Read the model definition and answer for the solid it produces. Units are mm, in the model's axes. Coordinates: 2 decimals unless noted, no trailing zeros. Loops run counter-clockwise (first coordinate to the right, second up) from the corner with the lowest first, then second, coordinate; pieces in that order, holes last.
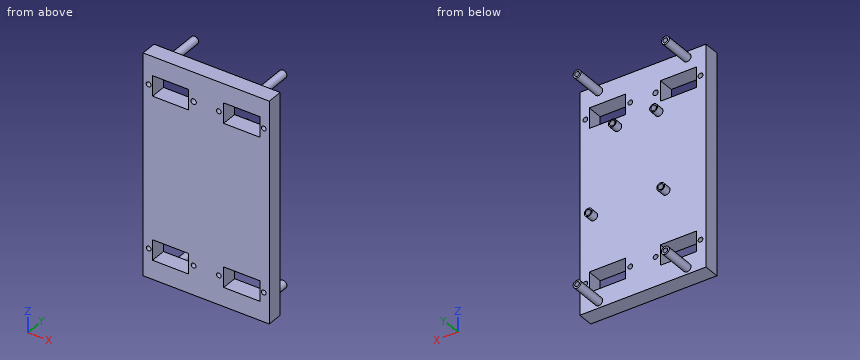
from build123d import *

# Parameters (mm, degrees)
SKETCH1_W           = 80
SKETCH1_H           = 140
BOSS_EXTRUDE1_DEPTH = 10
SKETCH4_W           = 22.9
SKETCH4_H           = 12.9
CUT_EXTRUDE2_DEPTH  = 162.554944214
SKETCH6_R           = 1.5
CUT_EXTRUDE4_DEPTH  = 162.554944214
SKETCH9_W           = 22.9
SKETCH9_H           = 12.9
CUT_EXTRUDE5_DEPTH  = 162.554944214
SKETCH13_R          = 2.5
BOSS_EXTRUDE2_DEPTH = 20
SKETCH14_R          = 1.5
CUT_EXTRUDE8_DEPTH  = 5
SKETCH15_R          = 2.5
BOSS_EXTRUDE3_DEPTH = 20
SKETCH16_R          = 1.5
CUT_EXTRUDE9_DEPTH  = 5
SKETCH17_R          = 1.567331153
SKETCH17_R_2        = 1.710433461
CUT_EXTRUDE10_DEPTH = 163.480768093
SKETCH24_R          = 2.5
BOSS_EXTRUDE5_DEPTH = 5
SKETCH26_R          = 1.8
CUT_EXTRUDE11_DEPTH = 5


with BuildPart() as part:
    # Sketch1 → Boss-Extrude1 (new body)
    with BuildSketch(Plane(origin=(0, 0, 0), x_dir=(1, 0, 0), z_dir=(0, 1, 0))):
        with Locations((-40, 70)):
            Rectangle(SKETCH1_W, SKETCH1_H)
    extrude(amount=BOSS_EXTRUDE1_DEPTH)

    # Sketch4 → Cut-Extrude2 (cut, through all)
    with BuildSketch(Plane(origin=(0, 10, 0), x_dir=(1, 0, 0), z_dir=(0, 1, 0))):
        with Locations((-17.45, 121.55)):
            Rectangle(SKETCH4_W, SKETCH4_H)
    cut_extrude2 = extrude(amount=-CUT_EXTRUDE2_DEPTH, mode=Mode.SUBTRACT)

    # Sketch6 → Cut-Extrude4 (cut, through all)
    with BuildSketch(Plane(origin=(0, 10, 0), x_dir=(1, 0, 0), z_dir=(0, 1, 0))):
        with Locations(Location((-3.5, 121.55, 0), (0, 0, 270))):
            Circle(SKETCH6_R)
        with Locations(Location((-32, 121.55, 0), (0, 0, 270))):
            Circle(SKETCH6_R)
    cut_extrude4 = extrude(amount=-CUT_EXTRUDE4_DEPTH, mode=Mode.SUBTRACT)

    # Mirror4: Cut-Extrude2, Cut-Extrude4 across plane
    add(cut_extrude2.mirror(Plane.XY.offset(-70)), mode=Mode.SUBTRACT)
    add(cut_extrude4.mirror(Plane.XY.offset(-70)), mode=Mode.SUBTRACT)

    # Mirror15: Cut-Extrude2, Cut-Extrude4 across plane
    add(cut_extrude2.mirror(Plane.ZY.offset(40)), mode=Mode.SUBTRACT)
    add(cut_extrude4.mirror(Plane.ZY.offset(40)), mode=Mode.SUBTRACT)

    # Sketch9 → Cut-Extrude5 (cut, through all)
    with BuildSketch(Plane(origin=(0, 10, 0), x_dir=(1, 0, 0), z_dir=(0, 1, 0))):
        with Locations((-62.55, 18.45)):
            Rectangle(SKETCH9_W, SKETCH9_H)
    extrude(amount=-CUT_EXTRUDE5_DEPTH, mode=Mode.SUBTRACT)

    # Sketch13 → Boss-Extrude2 (add)
    with BuildSketch(Plane(origin=(0, 10, 0), x_dir=(1, 0, 0), z_dir=(0, 1, 0))):
        with Locations(Location((-68, 136, 0), (0, 0, 270))):
            Circle(SKETCH13_R)
    boss_extrude2 = extrude(amount=BOSS_EXTRUDE2_DEPTH)

    # Sketch14 → Cut-Extrude8 (cut)
    with BuildSketch(Plane(origin=(0, 30, 0), x_dir=(1, 0, 0), z_dir=(0, 1, 0))):
        with Locations(Location((-68, 136, 0), (0, 0, 270))):
            Circle(SKETCH14_R)
    cut_extrude8 = extrude(amount=-CUT_EXTRUDE8_DEPTH, mode=Mode.SUBTRACT)

    # Sketch15 → Boss-Extrude3 (add)
    with BuildSketch(Plane(origin=(0, 10, 0), x_dir=(1, 0, 0), z_dir=(0, 1, 0))):
        with Locations(Location((-12, 136, 0), (0, 0, 270))):
            Circle(SKETCH15_R)
    boss_extrude3 = extrude(amount=BOSS_EXTRUDE3_DEPTH)

    # Sketch16 → Cut-Extrude9 (cut)
    with BuildSketch(Plane(origin=(0, 30, 0), x_dir=(1, 0, 0), z_dir=(0, 1, 0))):
        with Locations(Location((-12, 136, 0), (0, 0, 270))):
            Circle(SKETCH16_R)
    cut_extrude9 = extrude(amount=-CUT_EXTRUDE9_DEPTH, mode=Mode.SUBTRACT)

    # Mirror22: Boss-Extrude2, Cut-Extrude8, Boss-Extrude3, Cut-Extrude9 across plane
    add(boss_extrude2.mirror(Plane.XY.offset(-70)))
    add(cut_extrude8.mirror(Plane.XY.offset(-70)), mode=Mode.SUBTRACT)
    add(boss_extrude3.mirror(Plane.XY.offset(-70)))
    add(cut_extrude9.mirror(Plane.XY.offset(-70)), mode=Mode.SUBTRACT)

    # Sketch17 → Cut-Extrude10 (cut, through all)
    with BuildSketch(Plane(origin=(0, 10, 0), x_dir=(1, 0, 0), z_dir=(0, 1, 0))):
        with Locations(Location((-76.5, 18.45, 0), (0, 0, 270))):
            Circle(SKETCH17_R)
        with Locations(Location((-48, 18.45, 0), (0, 0, 270))):
            Circle(SKETCH17_R_2)
    extrude(amount=-CUT_EXTRUDE10_DEPTH, mode=Mode.SUBTRACT)

    # Sketch24 → Boss-Extrude5 (add)
    with BuildSketch(Plane(origin=(0, 10, 0), x_dir=(1, 0, 0), z_dir=(0, 1, 0))):
        with Locations(Location((-54.703909306, 82.704708795, 0), (0, 0, 270))):
            Circle(SKETCH24_R)
        with Locations(Location((-8.776377109, 81.387548885, 0), (0, 0, 270))):
            Circle(SKETCH24_R)
        with Locations(Location((-24.025346163, 31.067743918, 0), (0, 0, 270))):
            Circle(SKETCH24_R)
        with Locations(Location((-50.214312923, 31.502322072, 0), (0, 0, 270))):
            Circle(SKETCH24_R)
    extrude(amount=BOSS_EXTRUDE5_DEPTH)

    # Sketch26 → Cut-Extrude11 (cut)
    with BuildSketch(Plane(origin=(0, 15, 0), x_dir=(1, 0, 0), z_dir=(0, 1, 0))):
        with Locations(Location((-54.703909306, 82.704708795, 0), (0, 0, 270))):
            Circle(SKETCH26_R)
        with Locations(Location((-8.776377109, 81.387548885, 0), (0, 0, 270))):
            Circle(SKETCH26_R)
        with Locations(Location((-24.025346163, 31.067743918, 0), (0, 0, 270))):
            Circle(SKETCH26_R)
        with Locations(Location((-50.214312923, 31.502322072, 0), (0, 0, 270))):
            Circle(SKETCH26_R)
    extrude(amount=-CUT_EXTRUDE11_DEPTH, mode=Mode.SUBTRACT)


solid = part.part
Q1. A cutting plane is placed at A-A (z = -18.45). Give the vertices of the cut face in (x, y), then the cut area to 3 significant figures.
Findings below:
outline: (-80, 0) - (-78.07, 0) - (-78.07, 10) - (-80, 10) - close; (-74.93, 0) - (-74, 0) - (-74, 10) - (-74.93, 10) - close; (-51.1, 0) - (-49.71, 0) - (-49.71, 10) - (-51.1, 10) - close; (-46.29, 0) - (-33.5, 0) - (-33.5, 10) - (-46.29, 10) - close; (-30.5, 0) - (-28.9, 0) - (-28.9, 10) - (-30.5, 10) - close; (-6, 0) - (-5, 0) - (-5, 10) - (-6, 10) - close; (-2, 0) - (0, 0) - (0, 10) - (-2, 10) - close
area: 216 mm2
Q2. A cutting plane is placed at C-C (y = 6.5). Count the separate pieces of the cut face and the enclosed holes in it, then the cut area to 3 significant figures.
Findings below:
separate pieces: 1
enclosed holes: 12
area: 9,960 mm2
Q3. A cutting plane is placed at D-D (z = -118). Give the vertices of the cut face in (x, y).
Findings below:
outline: (-80, 0) - (-74, 0) - (-74, 10) - (-80, 10) - close; (-51.1, 0) - (-28.9, 0) - (-28.9, 10) - (-51.1, 10) - close; (-6, 0) - (0, 0) - (0, 10) - (-6, 10) - close
Q4. A cutting plane is placed at B-B (x = -68). Give the vertices of the cut face in (y, z).
Findings below:
outline: (0, -140) - (10, -140) - (10, -138.5) - (30, -138.5) - (30, -137.5) - (25, -137.5) - (25, -134.5) - (30, -134.5) - (30, -133.5) - (10, -133.5) - (10, -128) - (0, -128) - close; (0, -115.1) - (10, -115.1) - (10, -24.9) - (0, -24.9) - close; (0, -12) - (10, -12) - (10, -6.5) - (30, -6.5) - (30, -5.5) - (25, -5.5) - (25, -2.5) - (30, -2.5) - (30, -1.5) - (10, -1.5) - (10, 0) - (0, 0) - close
Q5. Flat-ended cylindrical pins translate along their axes: pin 1 Ø4 at (x, z) = (-32, -18.45) entering from +Y; pin 2 Ø1.5 at (x, z) = (-49.5, -32.5) entering from +Y. Find the tip coordinate at first contact, or state that the pin passes through.
Findings below:
pin 1: stops at y = 10
pin 2: stops at y = 15
Q6. Straight lines are drawn through the part: probe 1 along Z at (x, y) = (-69, 5.25); probe 2 along X at (y, z) = (5.25, -118); probe 3 along Z at (x, y) = (-67.5, 28.5). For each, find the intervals that lie inside material, in ascending order.
Findings below:
probe 1: z = -140 to -128, -115.1 to -24.9, -12 to 0
probe 2: x = -80 to -74, -51.1 to -28.9, -6 to 0
probe 3: z = -138.45 to -137.41, -134.59 to -133.55, -6.45 to -5.41, -2.59 to -1.55
